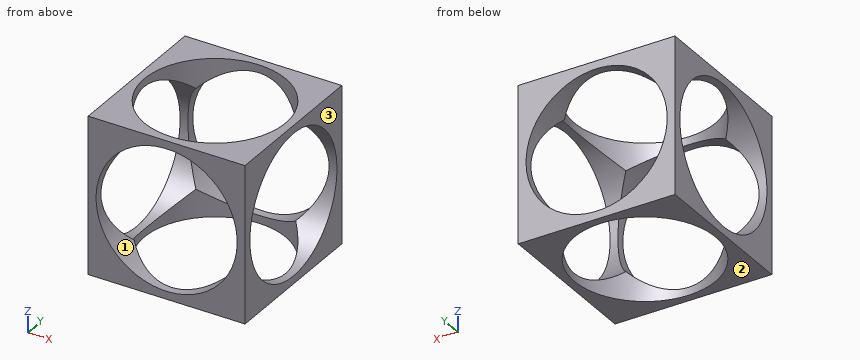
```python
from build123d import *

# Parameters (mm, degrees)
SKETCH1_W          = 100
SKETCH1_H          = 100
EXTRUDE1_DEPTH     = 100
SKETCH2_R          = 45
CUT_EXTRUDE1_DEPTH = 174.205080757
SKETCH4_R          = 45
CUT_EXTRUDE2_DEPTH = 174.205080757
SKETCH5_R          = 45
CUT_EXTRUDE3_DEPTH = 174.205080757


with BuildPart() as part:
    # Sketch1 → Extrude1 (new body)
    with BuildSketch(Plane.XY):
        with Locations((50, 50)):
            Rectangle(SKETCH1_W, SKETCH1_H)
    extrude(amount=EXTRUDE1_DEPTH)

    # Sketch2 → Cut-Extrude1 (cut, through all)
    with BuildSketch(Plane(origin=(0, 0, 0), x_dir=(0, 0, -1), z_dir=(1, 0, 0))):
        with Locations((-50, 50)):
            Circle(SKETCH2_R)
    extrude(amount=CUT_EXTRUDE1_DEPTH, mode=Mode.SUBTRACT)

    # Sketch4 → Cut-Extrude2 (cut, through all)
    with BuildSketch(Plane(origin=(100, 0, 0), x_dir=(1, 0, 0), z_dir=(0, 0, 1))):
        with Locations(Location((-50, 50, 0), (0, 0, 270))):
            Circle(SKETCH4_R)
    extrude(amount=CUT_EXTRUDE2_DEPTH, mode=Mode.SUBTRACT)

    # Sketch5 → Cut-Extrude3 (cut, through all)
    with BuildSketch(Plane(origin=(100, 0, 0), x_dir=(0, 0, -1), z_dir=(0, 1, 0))):
        with Locations(Location((-50, 50, 0), (0, 0, 45))):
            Circle(SKETCH5_R)
    extrude(amount=CUT_EXTRUDE3_DEPTH, mode=Mode.SUBTRACT)


solid = part.part
```
The listing builds one solid part. Answer for the finished solid, in the listing's coordinates (mm). Face numbers are marked on the shaded views. Give positions to 0.01 mm unless a question says otherwise; leave off trailing zeros. Order: outer loops, then holes, each group sorted by start corner. A loop starts at its lowest first (then second) coordinate and runs counter-clockwise, first axis right, second up.
Item 1: For a pull along Z with two mould halves and no side action, classify the marked faces 1, 2 and 3 as pulls with the +Z half, pulls with the -Z half, needs draft (parallel to the pull), parting line crosses it, or undercut.
From the geometry:
face 1: undercut
face 2: pulls with the -Z half
face 3: needs draft
Item 2: The part is cut by section C-C, the plane z = 12. Give the vertices of the cut face in (x, y), and give its area (3 significant figures).
From the geometry:
outline: (0, 0) - (25.9, 0) - (25.9, 12) arc R45 cw to (12, 25.9) - (0, 25.9) - close; (0, 74.1) - (12, 74.1) arc R45 cw to (25.9, 88) - (25.9, 100) - (0, 100) - close; (74.1, 0) - (100, 0) - (100, 25.9) - (88, 25.9) arc R45 cw to (74.1, 12) - close; (74.1, 88) arc R45 cw to (88, 74.1) - (100, 74.1) - (100, 100) - (74.1, 100) - close
area: 2,240 mm2
Item 3: Find the intervals of material crossed by probe 1 along Y at (x, z) = (50, 3.75); probe 2 along Z at (x, y) = (4, 34), in increasing order.
From the geometry:
probe 1: y = 0 to 5, 95 to 100
probe 2: z = 0 to 7.94, 92.06 to 100
Item 4: The part is cut by section D-D, the plane x = 10. Give the vertices of the cut face in (y, z).
From the geometry:
outline: (0, 0) - (29.38, 0) - (29.38, 10) arc R45 cw to (10, 29.38) - (0, 29.38) - close; (0, 70.62) - (10, 70.62) arc R45 cw to (29.38, 90) - (29.38, 100) - (0, 100) - close; (70.62, 0) - (100, 0) - (100, 29.38) - (90, 29.38) arc R45 cw to (70.62, 10) - close; (70.62, 90) arc R45 cw to (90, 70.62) - (100, 70.62) - (100, 100) - (70.62, 100) - close
Item 5: The part is cut by section A-A, the plane x = 50. Give the vertices of the cut face in (y, z), and give its area (3 significant figures).
From the geometry:
outline: (0, 0) - (5, 0) - (5, 5) - (0, 5) - close; (0, 95) - (5, 95) - (5, 100) - (0, 100) - close; (95, 0) - (100, 0) - (100, 5) - (95, 5) - close; (95, 95) - (100, 95) - (100, 100) - (95, 100) - close
area: 100 mm2
